```python
from build123d import *

# Parameters (mm, degrees)
EXTRUDE003_DEPTH                          = 5
EXTRUDE003_ONTO_SKETCH003_ROLL_ANGLE      = 90
EXTRUDE003_ONTO_SKETCH003_PLACEMENT_ANGLE = -90
EXTRUDE001_DEPTH                          = 9
EXTRUDE002_DEPTH                          = 2.5
SKETCH_R                                  = 1.75
EXTRUDE_DEPTH                             = 5
CHAMFER_SIZE                              = 2


with BuildPart() as extrude003:
    # Sketch003 as drawn → Extrude003 (new)
    with BuildSketch(Plane.XY):
        Polygon((-5, 16.5), (-5, 5), (0, 5), align=None)
    extrude(amount=-EXTRUDE003_DEPTH)


with BuildPart() as extrude003_1:
    # Extrude003 onto Sketch003 roll: moved
    add(extrude003.part.rotate(Axis((0, 0, 0), (1, 0, 0)), EXTRUDE003_ONTO_SKETCH003_ROLL_ANGLE))


with BuildPart() as extrude003_2:
    # Extrude003 onto Sketch003 placement: moved
    add(extrude003_1.part.moved(Location((5, 0, 0))).rotate(Axis((5, 0, 0), (0, 0, 1)), EXTRUDE003_ONTO_SKETCH003_PLACEMENT_ANGLE))


with BuildPart() as extrude003_3:
    # Extrude003 placement: moved
    add(extrude003_2.part.moved(Location((5, 0, 0))))


with BuildPart() as extrude003_mirrored:
    # mirror: instance of Extrude003
    add(extrude003_3.part.mirror(Plane(origin=(5, 5, 2), x_dir=(0.707107, 0.707107, 0), z_dir=(-0.707107, 0.707107, 0))))


with BuildPart() as extrude001:
    # Sketch001 (on Face12 of Extrude) → Extrude001 (new body)
    with BuildSketch(Plane.XY.offset(5)):
        Polygon((5, 30), (10, 30), (10, 10), (30, 10), (30, 5), (5, 5), align=None)
    extrude(amount=EXTRUDE001_DEPTH)


with BuildPart() as extrude002:
    # Sketch002 (on Face8 of Extrude001) → Extrude002 (new body)
    with BuildSketch(Plane.XY.offset(14)):
        Polygon((5, 30), (10, 30), (30, 10), (30, 5), (5, 5), align=None)
    extrude(amount=EXTRUDE002_DEPTH)


with BuildPart() as chamfer_body:
    # Sketch → Extrude (new body)
    with BuildSketch(Plane.XY):
        with BuildLine():
            Line((5, 30), (10, 30))
            Line((10, 10), (10, 30))
            Line((30, 10), (10, 10))
            Line((30, 10), (30, 5))
            Line((30, 5), (25, 0))
            Line((25, 0), (10, 0))
            ThreePointArc((0, 10), (-7.071068, -7.071068), (10, 0))
            Line((0, 10), (0, 25))
            Line((5, 30), (0, 25))
        make_face()
        Circle(SKETCH_R, mode=Mode.SUBTRACT)
    extrude(amount=EXTRUDE_DEPTH)

    # Fusion: union Extrude001, Extrude002
    add(extrude001.part)
    add(extrude002.part)

    # Fusion001: union Extrude003, Extrude003 (mirrored)
    add(extrude003_3.part)
    add(extrude003_mirrored.part)

    # Chamfer
    chamfer_edges = [chamfer_body.edges().sort_by_distance(p)[0] for p in [
        (5, 5, 10.75),
        (-1.75, 0, 5),
    ]]
    chamfer(chamfer_edges, length=CHAMFER_SIZE)


solid = chamfer_body.part
```
Here's how the part is built. I have some questions about the finished solid (model axes, mm). A direction names the side the tool comes from. Round coordinates to 2 decimals unless told otherwise and drop trailing zeros. Order: outer loops, then holes, each group sorted by start corner. A loop starts at its lowest first (then second) coordinate and runs counter-clockwise, first axis right, second up. Notation, with made-up numbers: M 89.25,65 L 132.25,65 A23 cw 132.25,90 Z; hole C 40,54 d9. An arc over 180 degrees is marked long. Use CSV: the item, a comma, the result in double quotes.
1) If we mould it in two halves opening along Y, with no side actions, what happens to faces 1 (the flat face through (21, 3, 5)), 2 (the cylindrical face through (1.617, -0.67, 1.479)), 3 (the flat face through (23, 5, 11))? For each: pulls with the +Y half, pulls with the -Y half, needs draft (parallel to the pull), parting line crosses it, or undercut.
Taken from the geometry:
face 1,"needs draft"
face 2,"undercut"
face 3,"pulls with the -Y half"
2) I want a section at B-B (x = 18). List the corners of the cut face in (y, z) for me.
Taken from the geometry:
outline,"M 0,0 L 10,0 L 10,14 L 22,14 L 22,16.5 L 5,16.5 L 5,5 L 0,5 Z"
3) I want a section at C-C (z = 10.75). List the corners of the cut face in (x, y) for me, then the cut area to 3 significant figures.
Taken from the geometry:
outline,"M 2.5,10 L 5,10 L 5,7 L 7,5 L 10,5 L 10,2.5 L 15,2.5 L 15,5 L 30,5 L 30,10 L 10,10 L 10,30 L 5,30 L 5,15 L 2.5,15 Z"
area,"248 mm^2"
4) I want a section at D-D (y = 11.5). List the corners of the cut face in (x, z) for me, then the cut area to 4 significant figures.
Taken from the geometry:
outline,"M 0,0 L 10,0 L 10,14 L 28.5,14 L 28.5,16.5 L 5,16.5 L 0,5 Z"
area,"182.5 mm^2"
5) I want a section at A-A (y = 26). List the corners of the cut face in (x, z) for me.
Taken from the geometry:
outline,"M 1,0 L 10,0 L 10,14 L 14,14 L 14,16.5 L 5,16.5 L 5,5 L 1,5 Z"
6) I need wall thicknesses on line 1 along Z through (x, y) = (19, 14); line 2 along X through (y, z) = (23.5, 15.5); line 3 along X through (y, z) = (12, 9). Which ranges of each line are inside material? Lowest first, please. Write a range as [from, to].
Taken from the geometry:
line 1,"[14, 16.5]"
line 2,"[5, 16.5]"
line 3,"[1.74, 10]"
7) I'm going to push flat-ended pins straight in: P1, Ø2, axis at x = 25, y = 15, coming from the -Z side; P2, Ø4, axis at x = 16.5, z = 7, coming from the +Y side; P3, Ø0.9, axis at x = 9, z = 8.5, coming from the -Y side. Where does each tip first touch, or does it pass through?
Taken from the geometry:
P1,"z = 14"
P2,"y = 10"
P3,"y = 5"
8) On a 3-axis mill with a long thin cutter (end or side, diameter ignored), from which of +Z, -Z, +X, -X, +Y, -Y can I reach the whole of each face in a straight line? I mean faces 4 (the flat face through (10, 4, 8)), 5 (the flat face through (16, 16, 14)), 6 (the flat face through (5, 22, 11)). Say none if no direction works.
Taken from the geometry:
face 4,"+Z, -X, -Y"
face 5,"-Z, +X, +Y"
face 6,"+Z, -X, +Y"
